Can you work these out from the model? Positions are in its coordinate system, mm. Round coordinates to 2 decimals unless told otherwise and drop trailing zeros. Loops run counter-clockwise (first coordinate to the right, second up) from the corner with the lowest first, then second, coordinate; pieces in that order, holes last.
(1) Will these pins go through, and if not, where does the flat tip stop? pin 1 Ø3 at (x, y) = (-75.5, 13.5) entering from -Z; pin 2 Ø3 at (x, y) = (2, 40) entering from -Z.
(2) I want a section at A-A on x = -80. Write out the boundary of the cut face in (y, z) (3 decimals).
(3) If I drill on line 1 along X through (y, z) = (10, 1.05); line 2 along Y through (x, z) = (2, 0.6); line 3 along Y through (x, z) = (-80.5, 0.1) (3 decimals), over which ranges is the centre line in solid material (lowest first)?
(4) I want a section at C-C on z = 0.45. Give the number of separate pieces and of enclosed holes in the cut face, plus the area to 3 significant figures.
(5) I want a section at B-B on x = 2. Write out the boundary of the cut face in (y, z), plus the area to 3 significant figures.
from build123d import *

# Parameters (mm, degrees)
MODEL_W            = 96
MODEL_H            = 46
MODEL_R            = 1.25
MODEL_R_2          = 2
MODEL_R_3          = 0.65
MODEL_R_4          = 1.2
MODEL_R_5          = 0.75
MODEL_R_6          = 3.375
MODEL_W_2          = 2.5
MODEL_H_2          = 2.5
MODEL_W_3          = 1.3
MODEL_H_3          = 1.3
MODEL_W_4          = 1.5
MODEL_H_4          = 1.5
MODEL_W_5          = 6.75
MODEL_H_5          = 6.75
BOSS_EXTRU_1_DEPTH = 1.6


with BuildPart() as part:
    # Model → Boss.-Extru.1 (new body)
    with BuildSketch(Plane.XY):
        with Locations((-43, 20)):
            Rectangle(MODEL_W, MODEL_H)
        with Locations((-58.928, 38.758)):
            Circle(MODEL_R, mode=Mode.SUBTRACT)
        with Locations((-57.404, 1.882)):
            Circle(MODEL_R, mode=Mode.SUBTRACT)
        with Locations((-88, 40)):
            Circle(MODEL_R_2, mode=Mode.SUBTRACT)
        with Locations((-88, 0)):
            Circle(MODEL_R_2, mode=Mode.SUBTRACT)
        with Locations((2, 0)):
            Circle(MODEL_R_2, mode=Mode.SUBTRACT)
        with Locations((2, 40)):
            Circle(MODEL_R_2, mode=Mode.SUBTRACT)
        with Locations((-7.112, 26.012)):
            Circle(MODEL_R, mode=Mode.SUBTRACT)
        with Locations((-7.112, 22.052)):
            Circle(MODEL_R, mode=Mode.SUBTRACT)
        with Locations((-7.112, 18.092)):
            Circle(MODEL_R, mode=Mode.SUBTRACT)
        with Locations((-7.112, 14.132)):
            Circle(MODEL_R, mode=Mode.SUBTRACT)
        with Locations((-7.112, 10.172)):
            Circle(MODEL_R, mode=Mode.SUBTRACT)
        with Locations((-18.542, 26.012)):
            Circle(MODEL_R, mode=Mode.SUBTRACT)
        with Locations((-18.542, 22.052)):
            Circle(MODEL_R, mode=Mode.SUBTRACT)
        with Locations((-18.542, 18.092)):
            Circle(MODEL_R, mode=Mode.SUBTRACT)
        with Locations((-18.542, 14.132)):
            Circle(MODEL_R, mode=Mode.SUBTRACT)
        with Locations((-18.542, 10.172)):
            Circle(MODEL_R, mode=Mode.SUBTRACT)
        with Locations((-29.972, 26.012)):
            Circle(MODEL_R, mode=Mode.SUBTRACT)
        with Locations((-29.972, 22.052)):
            Circle(MODEL_R, mode=Mode.SUBTRACT)
        with Locations((-29.972, 18.092)):
            Circle(MODEL_R, mode=Mode.SUBTRACT)
        with Locations((-29.972, 14.132)):
            Circle(MODEL_R, mode=Mode.SUBTRACT)
        with Locations((-29.972, 10.172)):
            Circle(MODEL_R, mode=Mode.SUBTRACT)
        with Locations((-36.068, 3.302)):
            Circle(MODEL_R_3, mode=Mode.SUBTRACT)
        with Locations((-33.528, 3.302)):
            Circle(MODEL_R_3, mode=Mode.SUBTRACT)
        with Locations((-21.59, 37.084)):
            Circle(MODEL_R_3, mode=Mode.SUBTRACT)
        with Locations((-19.05, 37.084)):
            Circle(MODEL_R_3, mode=Mode.SUBTRACT)
        with Locations((-36.322, 37.084)):
            Circle(MODEL_R_3, mode=Mode.SUBTRACT)
        with Locations((-33.782, 37.084)):
            Circle(MODEL_R_3, mode=Mode.SUBTRACT)
        with Locations((-63.492, 14.478)):
            Circle(MODEL_R_4, mode=Mode.SUBTRACT)
        with Locations((-37.092, 14.478)):
            Circle(MODEL_R_4, mode=Mode.SUBTRACT)
        with Locations((-63.492, 25.908)):
            Circle(MODEL_R_4, mode=Mode.SUBTRACT)
        with Locations((-37.092, 25.908)):
            Circle(MODEL_R_4, mode=Mode.SUBTRACT)
        with Locations((-75.398, 21.336)):
            Circle(MODEL_R_5, mode=Mode.SUBTRACT)
        with Locations((-75.398, 37.592)):
            Circle(MODEL_R_5, mode=Mode.SUBTRACT)
        with Locations((-71.44, 4.064)):
            Circle(MODEL_R_6, mode=Mode.SUBTRACT)
        with Locations((-71.186, 13.97)):
            Circle(MODEL_R_6, mode=Mode.SUBTRACT)
        with Locations((-70.932, 30.226)):
            Circle(MODEL_R_6, mode=Mode.SUBTRACT)
        with Locations((-58.928, 34.798)):
            Rectangle(MODEL_W_2, MODEL_H_2, mode=Mode.SUBTRACT)
        with Locations((-57.404, 5.842)):
            Rectangle(MODEL_W_2, MODEL_H_2, mode=Mode.SUBTRACT)
        with Locations((-7.112, 29.972)):
            Rectangle(MODEL_W_2, MODEL_H_2, mode=Mode.SUBTRACT)
        with Locations((-18.542, 29.972)):
            Rectangle(MODEL_W_2, MODEL_H_2, mode=Mode.SUBTRACT)
        with Locations((-29.972, 29.972)):
            Rectangle(MODEL_W_2, MODEL_H_2, mode=Mode.SUBTRACT)
        with Locations((-38.608, 3.302)):
            Rectangle(MODEL_W_3, MODEL_H_3, mode=Mode.SUBTRACT)
        with Locations((-24.13, 37.084)):
            Rectangle(MODEL_W_3, MODEL_H_3, mode=Mode.SUBTRACT)
        with Locations((-38.862, 37.084)):
            Rectangle(MODEL_W_3, MODEL_H_3, mode=Mode.SUBTRACT)
        with Locations((-72.898, 21.336)):
            Rectangle(MODEL_W_4, MODEL_H_4, mode=Mode.SUBTRACT)
        with Locations((-72.898, 37.592)):
            Rectangle(MODEL_W_4, MODEL_H_4, mode=Mode.SUBTRACT)
        with Locations((-78.74, 4.064)):
            Rectangle(MODEL_W_5, MODEL_H_5, mode=Mode.SUBTRACT)
        with Locations((-78.486, 13.97)):
            Rectangle(MODEL_W_5, MODEL_H_5, mode=Mode.SUBTRACT)
        with Locations((-78.232, 30.226)):
            Rectangle(MODEL_W_5, MODEL_H_5, mode=Mode.SUBTRACT)
    extrude(amount=BOSS_EXTRU_1_DEPTH)


solid = part.part
Filled sheet:
1. pin 1: stops at z = 0
1. pin 2: passes through
2. outline: (-3, 0) - (0.689, 0) - (0.689, 1.6) - (-3, 1.6) - close; (7.439, 0) - (10.595, 0) - (10.595, 1.6) - (7.439, 1.6) - close; (17.345, 0) - (26.851, 0) - (26.851, 1.6) - (17.345, 1.6) - close; (33.601, 0) - (43, 0) - (43, 1.6) - (33.601, 1.6) - close
3. line 1: x = -91 to -31.21, -28.73 to -19.78, -17.3 to -8.35, -5.87 to 5
3. line 2: y = -3 to -2, 2 to 38, 42 to 43
3. line 3: y = -3 to 0.689, 7.439 to 10.595, 17.345 to 26.851, 33.601 to 43
4. separate pieces: 1
4. enclosed holes: 49
4. area: 3,970 mm2
5. outline: (-3, 0) - (-2, 0) - (-2, 1.6) - (-3, 1.6) - close; (2, 0) - (38, 0) - (38, 1.6) - (2, 1.6) - close; (42, 0) - (43, 0) - (43, 1.6) - (42, 1.6) - close
5. area: 60.8 mm2
